Check sheet for the modelled part. Datum: model origin and axes. Units: mm. A direction names the side the tool comes from. Round coordinates to 2 decimals unless told otherwise and drop trailing zeros. Order: outer loops, then holes, each group sorted by start corner. A loop starts at its lowest first (then second) coordinate and runs counter-clockwise, first axis right, second up. Notation, with made-up numbers: M -13.75,-37 L 30.25,-37 A18 cw 30.25,-3 Z; hole C 88.5,-23.75 d9. An arc over 180 degrees is marked long. One line per item, written item: value. Start each with the question number.
(1) Access from +Z, -Z, +X, -X, +Y, -Y to the whole of each face (thin tool, end or side, straight path). Record for faces 4 (the face through (-24, -41, 4)), 5 (the face through (0, -45, -7.3)), 6 (the face through (-1.172, -0.354, 8.923)).
(2) Cross-section at A-A, the plane y = -13. Enter the section's corners in (x, z).
(3) Depth check by flat-ended pin: pin 1 Ø2 at (y, z) = (-33, -20.5) entering from +X; pin 2 Ø1 at (x, z) = (-12, 19) entering from -Y; pin 3 Ø12.5 at (x, z) = (0, 0) entering from +Y; pin 4 Ø4 at (y, z) = (-14.5, 9.5) entering from -X. Enter the tip coordinate at first touch or a pass-through.
(4) Release check for a two-part mould opening along Z. For faces 1 (the face through (-12, -2, -11)), 2 (the face through (14.246, -22.241, 22.345)), 3 (the face through (6.466, -22.185, -2.681)) record: released by +Z, released by -Z, zero draft, split by the parting line, or undercut.
(5) Thickness scan on L1, parallel to Z at x = 0, y = -33; L2, parallel to Y at x = -22, z = -10.5; L3, parallel to Z at x = -3.5, y = -34. Record the ranges inside material, lowest first.
from build123d import *

# Parameters (mm, degrees)
F0_R      = 9
F0_R_2    = 7
F1_DEPTH  = 45
F3_R      = 16
F3_R_2    = 9
F4_DEPTH  = 35
F6_R      = 18
F6_R_2    = 16
F7_DEPTH  = 41
F9_R      = 26.5
F9_R_2    = 24
F10_DEPTH = 37
F12_R     = 24
F12_R_2   = 18
F13_DEPTH = 33


# Not quite as in the source:
# - a fillet or chamfer that OpenCascade refuses, or shapes differently, is made with other operations: its cross-section is extruded or revolved along the edge and cut away or added


with BuildPart() as f1:
    # F0 (on Front) → F1 (new body)
    with BuildSketch(Plane.XZ):
        Circle(F0_R)
        Circle(F0_R_2, mode=Mode.SUBTRACT)
    extrude(amount=F1_DEPTH)

    # F3 (on offset) → F4 (join)
    with BuildSketch(Plane.XZ.offset(5)):
        Circle(F3_R)
        Circle(F3_R_2, mode=Mode.SUBTRACT)
    extrude(amount=F4_DEPTH)

    # F6 (on offset) → F7 (join)
    with BuildSketch(Plane.XZ.offset(2)):
        Circle(F6_R)
        Circle(F6_R_2, mode=Mode.SUBTRACT)
    extrude(amount=F7_DEPTH)



with BuildPart() as f10:
    # F9 (on offset) → F10 (new body)
    with BuildSketch(Plane.XZ.offset(4)):
        Circle(F9_R)
        Circle(F9_R_2, mode=Mode.SUBTRACT)
    extrude(amount=F10_DEPTH)


with BuildPart() as f1_1:
    add(f1.part)

    add(f10.part)  # F13 merges F10
    # F12 (on offset) → F13 (join)
    with BuildSketch(Plane.XZ.offset(6)):
        Circle(F12_R)
        Circle(F12_R_2, mode=Mode.SUBTRACT)
    extrude(amount=F13_DEPTH)

    # F14: fillet of radius 5 on 2 edges, made by hand

    # F14_s1 → F14_t2 (revolve)
    with BuildSketch(Plane.XY):
        with BuildLine():
            ThreePointArc((16, -43), (14.1560370926, -40.8166998673), (11.417424305, -40))
            Line((11.417424305, -40), (16, -40))
            Line((16, -40), (16, -43))
        make_face()
    revolve(axis=Axis((0, -40, 0), (0, -1, 0)))

    # F14_s3 → F14_t4 (revolve)
    with BuildSketch(Plane.XY):
        with BuildLine():
            ThreePointArc((24, -41), (22.2360679775, -39.527864045), (20, -39))
            Line((20, -39), (24, -39))
            Line((24, -39), (24, -41))
        make_face()
    revolve(axis=Axis((0, -39, 0), (0, -1, 0)))

    # F15: fillet of radius 5 on 2 edges, made by hand

    # F15_s1 → F15_t2 (revolve)
    with BuildSketch(Plane.XY):
        with BuildLine():
            ThreePointArc((11.417424305, -40), (9.6461006859, -41.8230248202), (9, -44.2813902858))
            Line((9, -44.2813902858), (9, -40))
            Line((9, -40), (11.417424305, -40))
        make_face()
    revolve(axis=Axis((0, -40, 0), (0, -1, 0)))

    # F15_s3 → F15_t4 (revolve)
    with BuildSketch(Plane.XY):
        with BuildLine():
            ThreePointArc((20, -39), (18.527864045, -40.7639320225), (18, -43))
            Line((18, -43), (18, -39))
            Line((18, -39), (20, -39))
        make_face()
    revolve(axis=Axis((0, -39, 0), (0, -1, 0)))

    # F16: fillet of radius 5 on 2 edges, made by hand

    # F16_s1 → F16_t2 (revolve)
    with BuildSketch(Plane.XY):
        with BuildLine():
            ThreePointArc((16, -2), (14.1560370926, -4.1833001327), (11.417424305, -5))
            Line((11.417424305, -5), (16, -5))
            Line((16, -5), (16, -2))
        make_face()
    revolve(axis=Axis((0, -5, 0), (0, -1, 0)))

    # F16_s3 → F16_t4 (revolve)
    with BuildSketch(Plane.XY):
        with BuildLine():
            ThreePointArc((24, -4), (22.2360679775, -5.472135955), (20, -6))
            Line((20, -6), (24, -6))
            Line((24, -6), (24, -4))
        make_face()
    revolve(axis=Axis((0, -6, 0), (0, -1, 0)))

    # F17: fillet of radius 5 on 2 edges, made by hand

    # F17_s1 → F17_t2 (revolve)
    with BuildSketch(Plane.XY):
        with BuildLine():
            ThreePointArc((11.417424305, -5), (9.6461006859, -3.1769751798), (9, -0.7186097142))
            Line((9, -0.7186097142), (9, -5))
            Line((9, -5), (11.417424305, -5))
        make_face()
    revolve(axis=Axis((0, -5, 0), (0, -1, 0)))

    # F17_s3 → F17_t4 (revolve)
    with BuildSketch(Plane.XY):
        with BuildLine():
            ThreePointArc((20, -6), (18.527864045, -4.2360679775), (18, -2))
            Line((18, -2), (18, -6))
            Line((18, -6), (20, -6))
        make_face()
    revolve(axis=Axis((0, -6, 0), (0, -1, 0)))


solid = f1_1.part
Values found:
1. face 4: -Y
1. face 5: +Z, -Z, +X, -X, -Y
1. face 6: +Y
2. outline: C 0,0 d53; hole C 0,0 d14
3. pin 1: x = 17.94
3. pin 2: y = -39.98
3. pin 3: through
3. pin 4: x = -25.42
4. face 1: zero draft
4. face 2: split by the parting line
4. face 3: undercut
5. L1: -26.5 to -7, 7 to 26.5
5. L2: -41 to -4
5. L3: -26.27 to -6.06, 6.06 to 26.27
